The listing builds one solid part. Answer for the finished solid, in the listing's coordinates (mm). A direction names the side the tool comes from. Coordinates: 2 decimals unless noted, no trailing zeros. Order: outer loops, then holes, each group sorted by start corner. A loop starts at its lowest first (then second) coordinate and runs counter-clockwise, first axis right, second up.
```python
from build123d import *

# Parameters (mm, degrees)
SKETCH_1_W          = 375
SKETCH_1_H          = 260
EXTRUDE_1_DEPTH     = 115
SHELL_1_T           = -5
SKETCH_2_R          = 1.5
CUT_EXTRUDE_1_DEPTH = 5


with BuildPart() as part:
    # Эскиз1 → Бобышка-Вытянуть1 (new body)
    with BuildSketch(Plane(origin=(0, 0, 0), x_dir=(1, 0, 0), z_dir=(0, 1, 0))):
        Rectangle(SKETCH_1_W, SKETCH_1_H)
    extrude(amount=EXTRUDE_1_DEPTH)

    # Оболочка1
    shell_1_openings = [part.faces().sort_by_distance(p)[0] for p in [
        (0, 115, 0),
    ]]
    offset(amount=SHELL_1_T, openings=shell_1_openings, kind=Kind.INTERSECTION)

    # Эскиз2 → Вырез-Вытянуть1 (cut)
    with BuildSketch(Plane(origin=(0, 0, -130), x_dir=(-1, 0, 0), z_dir=(0, 0, -1))):
        with Locations((-34.5, 60)):
            Circle(SKETCH_2_R)
        with Locations(Location((-1.1, 60, 0), (0, 0, 180))):
            Circle(SKETCH_2_R)
        with Locations((9.9, 60)):
            Circle(SKETCH_2_R)
        with Locations(Location((43.3, 60, 0), (0, 0, 180))):
            Circle(SKETCH_2_R)
        with Locations((-34.5, 40)):
            Circle(SKETCH_2_R)
        with Locations(Location((-1.1, 40, 0), (0, 0, 180))):
            Circle(SKETCH_2_R)
        with Locations((9.9, 40)):
            Circle(SKETCH_2_R)
        with Locations(Location((43.3, 40, 0), (0, 0, 180))):
            Circle(SKETCH_2_R)
        with Locations((-94.2, 40.5)):
            Circle(SKETCH_2_R)
        with Locations((-94.2, 79.5)):
            Circle(SKETCH_2_R)
        with BuildLine():
            Line((-31.3, 57), (-29.9529459, 64.184288535))
            ThreePointArc((-29.9529459, 64.184288535), (-29.60870955, 64.769509108), (-28.970073713, 65))
            Line((-28.970073713, 65), (-6.629926287, 65))
            ThreePointArc((-6.629926287, 65), (-5.99129045, 64.769509108), (-5.6470541, 64.184288535))
            Line((-5.6470541, 64.184288535), (-4.317127813, 57.091348336))
            ThreePointArc((-4.317127813, 57.091348336), (-4.30429116, 56.999601179), (-4.3, 56.907059801))
            Line((-4.3, 56.907059801), (-4.3, 56))
            ThreePointArc((-4.3, 56), (-4.592893219, 55.292893219), (-5.3, 55))
            Line((-5.3, 55), (-30.3, 55))
            ThreePointArc((-30.3, 55), (-31.007106781, 55.292893219), (-31.3, 56))
            Line((-31.3, 56), (-31.3, 57))
        make_face()
        with BuildLine():
            Line((13.1, 57), (14.4470541, 64.184288535))
            ThreePointArc((14.4470541, 64.184288535), (14.79129045, 64.769509108), (15.429926287, 65))
            Line((15.429926287, 65), (37.770073713, 65))
            ThreePointArc((37.770073713, 65), (38.40870955, 64.769509108), (38.7529459, 64.184288535))
            Line((38.7529459, 64.184288535), (40.082872187, 57.091348336))
            ThreePointArc((40.082872187, 57.091348336), (40.09570884, 56.999601179), (40.1, 56.907059801))
            Line((40.1, 56.907059801), (40.1, 56))
            ThreePointArc((40.1, 56), (39.807106781, 55.292893219), (39.1, 55))
            Line((39.1, 55), (14.1, 55))
            ThreePointArc((14.1, 55), (13.392893219, 55.292893219), (13.1, 56))
            Line((13.1, 56), (13.1, 57))
        make_face()
        with BuildLine():
            Line((-31.3, 37), (-29.9529459, 44.184288535))
            ThreePointArc((-29.9529459, 44.184288535), (-29.60870955, 44.769509108), (-28.970073713, 45))
            Line((-28.970073713, 45), (-6.629926287, 45))
            ThreePointArc((-6.629926287, 45), (-5.99129045, 44.769509108), (-5.6470541, 44.184288535))
            Line((-5.6470541, 44.184288535), (-4.317127813, 37.091348336))
            ThreePointArc((-4.317127813, 37.091348336), (-4.30429116, 36.999601179), (-4.3, 36.907059801))
            Line((-4.3, 36.907059801), (-4.3, 36))
            ThreePointArc((-4.3, 36), (-4.592893219, 35.292893219), (-5.3, 35))
            Line((-5.3, 35), (-30.3, 35))
            ThreePointArc((-30.3, 35), (-31.007106781, 35.292893219), (-31.3, 36))
            Line((-31.3, 36), (-31.3, 37))
        make_face()
        with BuildLine():
            Line((13.1, 37), (14.4470541, 44.184288535))
            ThreePointArc((14.4470541, 44.184288535), (14.79129045, 44.769509108), (15.429926287, 45))
            Line((15.429926287, 45), (37.770073713, 45))
            ThreePointArc((37.770073713, 45), (38.40870955, 44.769509108), (38.7529459, 44.184288535))
            Line((38.7529459, 44.184288535), (40.082872187, 37.091348336))
            ThreePointArc((40.082872187, 37.091348336), (40.09570884, 36.999601179), (40.1, 36.907059801))
            Line((40.1, 36.907059801), (40.1, 36))
            ThreePointArc((40.1, 36), (39.807106781, 35.292893219), (39.1, 35))
            Line((39.1, 35), (14.1, 35))
            ThreePointArc((14.1, 35), (13.392893219, 35.292893219), (13.1, 36))
            Line((13.1, 36), (13.1, 37))
        make_face()
        with BuildLine():
            Line((-113.1, 46.6), (-71.9, 46.6))
            ThreePointArc((-71.9, 46.6), (-71.192893219, 46.892893219), (-70.9, 47.6))
            Line((-70.9, 47.6), (-70.9, 72.4))
            ThreePointArc((-70.9, 72.4), (-71.192893219, 73.107106781), (-71.9, 73.4))
            Line((-71.9, 73.4), (-113.1, 73.4))
            Line((-113.1, 73.4), (-117.5, 69))
            Line((-117.5, 69), (-117.5, 51))
            Line((-117.5, 51), (-113.1, 46.6))
        make_face()
    extrude(amount=-CUT_EXTRUDE_1_DEPTH, mode=Mode.SUBTRACT)


solid = part.part
```
1) For faces 1 (the flat face through (182.5, 59, 2)), 2 (the flat face through (-1, 115, -126)), determine the directions among +Z, -Z, +X, -X, +Y, -Y from which every point of the face is accessible in a straight line to the end or side of a thin tool.
2) Straight lines are drawn through the part: probe 1 along Y at (x, z) = (94, -129); probe 2 along Y at (x, z) = (1.1, -128.9); probe 3 along X at (y, z) = (53, -107). For each, find the intervals that lie inside material, in ascending order.
3) A cutting plane is placed at C-C, the plane y = 31. Write down the section's boundary in (x, z), plus the area to 3 significant figures.
4) A cutting plane is placed at A-A, the plane x = -69. Write down the section's boundary in (y, z).
5) The mould has two halves that part along X. Classify faces 3 (the flat face through (187.5, 57, 2)), 4 (the flat face through (-182.5, 59, 2)), 5 (the flat face through (-3, 57, -130)): released by +X, released by -X, zero draft, split by the parting line, or undercut.
6) A cutting plane is placed at B-B, the plane z = 29. Write down the section's boundary in (x, y), plus the area to 4 significant figures.
7) Each of these flat-tipped pins is pushed along its axis until it touches: P1, Ø1, axis at x = -110, z = -27, coming from the +Y side; P2, Ø2.5, axis at x = 34.5, y = 60, coming from the -Z side. Where does it stop, or does it pass through?
Working result:
1. face 1: +Y
1. face 2: +Z, -Z, +X, -X, +Y
2. probe 1: y = 0 to 39.01, 41.99 to 46.6, 73.4 to 78.01, 80.99 to 115
2. probe 2: y = 0 to 38.5, 41.5 to 58.5, 61.5 to 115
2. probe 3: x = -187.5 to -182.5, 182.5 to 187.5
3. outline: (-187.5, -130) - (187.5, -130) - (187.5, 130) - (-187.5, 130) - close; hole (-182.5, -125) - (182.5, -125) - (182.5, 125) - (-182.5, 125) - close
3. area: 6,250 mm2
4. outline: (0, -130) - (115, -130) - (115, -125) - (5, -125) - (5, 125) - (115, 125) - (115, 130) - (0, 130) - close
5. face 3: released by +X
5. face 4: undercut
5. face 5: zero draft
6. outline: (-187.5, 0) - (187.5, 0) - (187.5, 115) - (182.5, 115) - (182.5, 5) - (-182.5, 5) - (-182.5, 115) - (-187.5, 115) - close
6. area: 2,975 mm2
7. P1: stops at y = 5
7. P2: stops at z = 125
